from build123d import *

# Parameters (mm, degrees)
F0_R     = 76.2
F0_R_2   = 3.175
F1_DEPTH = 19.05
F3_DEPTH = 6.35
F4_W     = 31.75
F4_H     = 3.175
F5_DEPTH = 3.175
F6_W     = 6.35
F6_H     = 79.386771
F7_DEPTH = 5.08


with BuildPart() as f1:
    # F0 (on Top) → F1 (new body)
    with BuildSketch(Plane.XY):
        Circle(F0_R)
        Circle(F0_R_2, mode=Mode.SUBTRACT)
    extrude(amount=F1_DEPTH)

    # F2 (on face) → F3 (cut)
    with BuildSketch(Plane.XY.offset(19.05)):
        Polygon((9.652, 39.966119), (-9.652, 39.966119), (-53.975, -29.675636), (53.975, -29.675636), align=None)
    extrude(amount=-F3_DEPTH, mode=Mode.SUBTRACT)

    # F4 (on face) → F5 (cut)
    with BuildSketch(Plane.XY.offset(19.05)):
        with Locations((0, -38.654536)):
            Rectangle(F4_W, F4_H)
        with Locations((0, -45.004536)):
            Rectangle(F4_W, F4_H)
        with Locations((0, -51.354536)):
            Rectangle(F4_W, F4_H)
        with Locations((0, -57.704536)):
            Rectangle(F4_W, F4_H)
        with Locations((0, -64.054536)):
            Rectangle(F4_W, F4_H)
        Polygon((46.16054, 44.984321), (62.03554, 17.488014), (64.785171, 19.075514), (48.910171, 46.571821), align=None)
        Polygon((40.038495, 4.788014), (42.788126, 6.375514), (26.913126, 33.871821), (24.163495, 32.284321), align=None)
        Polygon((59.28591, 15.900514), (43.41091, 43.396821), (40.661279, 41.809321), (56.536279, 14.313014), align=None)
        Polygon((32.412387, 37.046821), (29.662757, 35.459321), (45.537757, 7.963014), (48.287387, 9.550514), align=None)
        Polygon((35.162018, 38.634321), (51.037018, 11.138014), (53.786649, 12.725514), (37.911649, 40.221821), align=None)
        Polygon((-62.037835, 17.48669), (-46.162835, 44.982996), (-48.912466, 46.570496), (-64.787466, 19.07419), align=None)
        Polygon((-24.16579, 32.282996), (-26.91542, 33.870496), (-42.79042, 6.37419), (-40.04079, 4.78669), align=None)
        Polygon((-43.413204, 43.395496), (-59.288204, 15.89919), (-56.538574, 14.31169), (-40.663574, 41.807996), align=None)
        Polygon((-48.289682, 9.54919), (-45.540051, 7.96169), (-29.665051, 35.457996), (-32.414682, 37.045496), align=None)
        Polygon((-51.039312, 11.13669), (-35.164312, 38.632996), (-37.913943, 40.220496), (-53.788943, 12.72419), align=None)
    extrude(amount=-F5_DEPTH, mode=Mode.SUBTRACT)

    # F6 (on face) → F7 (cut)
    with BuildSketch(Plane(origin=(0, 0, 0), x_dir=(1, 0, 0), z_dir=(0, 0, -1))):
        with Locations((0, 39.693385)):
            Rectangle(F6_W, F6_H)
    extrude(amount=-F7_DEPTH, mode=Mode.SUBTRACT)


solid = f1.part
Geometry: final body of the model. Coordinates: model frame, mm. A direction names the side the tool comes from. Give positions to 0.01 mm unless a question says otherwise; leave off trailing zeros. Loops run counter-clockwise (first coordinate to the right, second up) from the corner with the lowest first, then second, coordinate; pieces in that order, holes last. Notation, with made-up numbers: (-36, 61.25) -> (6, 61.25) arc R19 ccw to (6, 68.25) -> close; hole circle Ø4 at (-2, 62). An arc over 180 degrees is marked (long way). Put each result on its own line as item: value.
1. Cut plane D-D (y = 49). Return the cut outline in (x, z), plus the area to 3 significant figures.
Taken from the geometry:
outline: (-58.36, 0) -> (58.36, 0) -> (58.36, 19.05) -> (-58.36, 19.05) -> close
area: 2,220 mm2
2. Pull-direction query (X, two-part tool) for faces 1 (the cylindrical face through (-60.47, -46.367, 9.392)), 2 (the flat face through (45.96, 26.28, 17.48)); classes: released by +X, released by -X, zero draft, split by the parting line, or undercut.
Taken from the geometry:
face 1: split by the parting line
face 2: undercut
3. Ray query, line 1 along X through (y, z) = (0, 5.25) (3 decimals); line 2 along Z through (x, y) = (13, -25). Return the intervals inside material, ascending. Write a range as [from, to].
Taken from the geometry:
line 1: x = [-76.2, -3.175], [3.175, 76.2]
line 2: z = [0, 12.7]
4. Set-up query: faces 3 (the flat face through (3.175, -38, 3)), 4 (the flat face through (-1, -10, 12.7)). Return all of +Z, -Z, +X, -X, +Y, -Y with unobstructed straight access to the full face (end or side cutting, diameter ignored); none if empty.
Taken from the geometry:
face 3: -Z, -Y
face 4: +Z
5. Cut plane C-C (y = -14). Return the cut outline in (x, z) (3 decimals), plus the area to 3 significant figures.
Taken from the geometry:
outline: (-74.903, 0) -> (-3.175, 0) -> (-3.175, 5.08) -> (3.175, 5.08) -> (3.175, 0) -> (74.903, 0) -> (74.903, 19.05) -> (43.998, 19.05) -> (43.998, 12.7) -> (-43.998, 12.7) -> (-43.998, 19.05) -> (-74.903, 19.05) -> close
area: 2,260 mm2
6. Cut plane B-B (z = 7.25). Return the cut outline in (x, y) (3 decimals).
Taken from the geometry:
outline: circle Ø152.4 at (0, 0); hole circle Ø6.35 at (0, 0)
7. Pin query (flat end, axial travel): P1, Ø1, axis at y = -64.5, z = 17, coming from the -X side; P2, Ø5, axis at x = -9.5, z = 12, coming from the +Y side; P3, Ø1.5, axis at y = -48.5, z = 3.5, coming from the +X side; P4, Ø15, axis at x = -41, y = 32, coming from the +Z side. Return the tip coordinate at first contact, or that it passes through.
Taken from the geometry:
P1: stops at x = -41.36
P2: stops at y = 75.88
P3: stops at x = 59.38
P4: stops at z = 19.05
